Source: CAD feature listing. Evaluate the final solid. Frame: model axes, mm. Round coordinates to 2 decimals unless told otherwise and drop trailing zeros. Loops run counter-clockwise (first coordinate to the right, second up) from the corner with the lowest first, then second, coordinate; pieces in that order, holes last. Notation, with made-up numbers: (17.5, 88.25) -> (41.5, 88.25) arc R13 cw to (41.5, 103.25) -> close; hole circle Ø10 at (32, 88.25). An arc over 180 degrees is marked (long way). Put each result on its own line as item: value. Start each with the question number.
1. Cut plane D-D (x = -43). Return the cut outline in (y, z), then the cut area to 3 significant figures.
2. Cut plane A-A (x = 65). Return the cut outline in (y, z), then the cut area to 3 significant figures.
3. Material intervals for L1, parallel to Z at x = 145, y = 325.6; L2, parallel to Z at x = -160.5, y = 325.05; L3, parallel to X at y = 326.3, z = -124.5, sorted ascending.
4. Contact query for flat-ended pins moving along their axis: pin 1 (3 mm diameter, centred on y = 323.5, z = -103.5, fed in from +X); pin 2 (3 mm diameter, centred on y = 325, z = -21, fed in from -X); pin 3 (1.8 mm diameter, centred on x = 54.5, y = 327, fed in from +Z). Output: stop coordinate, or through.
5. Cut plane C-C (y = 327.05). Return the cut outline in (x, z), then the cut area to 3 significant figures.
6. Cut plane B-B (z = 23). Return the cut outline in (x, y).
```python
from build123d import *

# Parameters (mm, degrees)
BOSS_EXTRUDE1_DEPTH = 6


with BuildPart() as part:
    # Sketch1 → Boss-Extrude1 (new body)
    with BuildSketch(Plane.XZ.offset(-323)):
        with BuildLine():
            Line((-52.025054896, -21.507337011), (-195.6, -21.507337011))
            ThreePointArc((-195.6, -21.507337011), (-199.838234915, -19.754378899), (-201.599987073, -15.519791945))
            Line((-201.599987073, -15.519791945), (-201.900014866, 129.014323174))
            ThreePointArc((-201.900014866, 129.014323174), (-208.810742902, 135.899991637), (-215.699996282, 128.992837374))
            Line((-215.699996282, 128.992837374), (-215.399996282, -160.007162626))
            ThreePointArc((-215.399996282, -160.007162626), (-213.376503762, -164.881568504), (-208.5, -166.9))
            Line((-208.5, -166.9), (208.8, -166.9))
            ThreePointArc((208.8, -166.9), (213.684597243, -164.873469993), (215.699982056, -159.984263701))
            Line((215.699982056, -159.984263701), (215.399982056, -28.441600712))
            ThreePointArc((215.399982056, -28.441600712), (213.373469993, -23.572739768), (208.5, -21.557337011))
            Line((208.5, -21.557337011), (3.974945104, -21.557337011))
            Line((3.974945104, -21.557337011), (3.974945104, -23.057337011))
            Line((3.974945104, -23.057337011), (208.5, -23.057337011))
            ThreePointArc((208.5, -23.057337011), (212.314019994, -24.634608733), (213.899985957, -28.445021647))
            Line((213.899985957, -28.445021647), (214.199985957, -159.987684636))
            ThreePointArc((214.199985957, -159.987684636), (212.622728277, -163.814019994), (208.8, -165.4))
            Line((208.8, -165.4), (-208.5, -165.4))
            ThreePointArc((-208.5, -165.4), (-212.316394249, -163.82035796), (-213.899997091, -160.005605533))
            Line((-213.899997091, -160.005605533), (-214.199997091, 128.994394467))
            ThreePointArc((-214.199997091, 128.994394467), (-208.808407488, 134.399993455), (-203.400011634, 129.011209441))
            Line((-203.400011634, 129.011209441), (-203.099983841, -15.522905679))
            ThreePointArc((-203.099983841, -15.522905679), (-200.897793644, -20.816139371), (-195.6, -23.007337011))
            Line((-195.6, -23.007337011), (-52.025054896, -23.007337011))
            Line((-52.025054896, -23.007337011), (-52.025054896, -21.507337011))
        make_face()
    extrude(amount=-BOSS_EXTRUDE1_DEPTH)


solid = part.part
```
Solution:
1. outline: (323, -166.9) -> (329, -166.9) -> (329, -165.4) -> (323, -165.4) -> close
1. area: 9.00 mm^2
2. outline: (323, -166.9) -> (329, -166.9) -> (329, -165.4) -> (323, -165.4) -> close; (323, -23.06) -> (329, -23.06) -> (329, -21.56) -> (323, -21.56) -> close
2. area: 18.0 mm^2
3. L1: z = -166.9 to -165.4, -23.06 to -21.56
3. L2: z = -166.9 to -165.4, -23.01 to -21.51
3. L3: x = -215.44 to -213.94, 214.12 to 215.62
4. pin 1: stops at x = 215.57
4. pin 2: stops at x = -215.55
4. pin 3: stops at z = -21.56
5. outline: (-215.7, 128.99) -> (-215.4, -160.01) arc R6.9 ccw to (-208.5, -166.9) -> (208.8, -166.9) arc R6.9 ccw to (215.7, -159.98) -> (215.4, -28.44) arc R6.9 ccw to (208.5, -21.56) -> (3.97, -21.56) -> (3.97, -23.06) -> (208.5, -23.06) arc R5.4 cw to (213.9, -28.45) -> (214.2, -159.99) arc R5.4 cw to (208.8, -165.4) -> (-208.5, -165.4) arc R5.4 cw to (-213.9, -160.01) -> (-214.2, 128.99) arc R5.4 cw to (-203.4, 129.01) -> (-203.1, -15.52) arc R7.5 ccw to (-195.6, -23.01) -> (-52.03, -23.01) -> (-52.03, -21.51) -> (-195.6, -21.51) arc R6 cw to (-201.6, -15.52) -> (-201.9, 129.01) arc R6.9 ccw to start
5. area: 2,080 mm^2
6. outline: (-215.59, 323) -> (-214.09, 323) -> (-214.09, 329) -> (-215.59, 329) -> close; (-203.18, 323) -> (-201.68, 323) -> (-201.68, 329) -> (-203.18, 329) -> close
